from build123d import *

# Parameters (mm, degrees)
SKETCH251_AS_DRAWN_R                 = 1
EXTRUDE052_DEPTH                     = 1
EXTRUDE052_ONTO_SKETCH251_ROLL_ANGLE = 90
SKETCH249_AS_DRAWN_R                 = 2
EXTRUDE051_DEPTH                     = 1
EXTRUDE051_ONTO_SKETCH249_ROLL_ANGLE = 90
EXTRUDE047_DEPTH                     = 31
EXTRUDE047_ONTO_SKETCH246_ROLL_ANGLE = 90
CHAMFER_SIZE                         = 1
EXTRUDE046_DEPTH                     = 32
EXTRUDE046_ONTO_SKETCH244_ROLL_ANGLE = 90
FILLET_R                             = 1
SKETCH248_AS_DRAWN_R                 = 2
EXTRUDE050_DEPTH                     = 2
EXTRUDE050_ONTO_SKETCH248_ROLL_ANGLE = 90
SKETCH247_AS_DRAWN_R                 = 3
EXTRUDE049_DEPTH                     = 2
EXTRUDE049_ONTO_SKETCH247_ROLL_ANGLE = 90
FILLET001_R                          = 0.5


with BuildPart() as extrude052:
    # Sketch251 as drawn → Extrude052 (new)
    with BuildSketch(Plane.XY):
        with Locations((4.5, 0)):
            Circle(SKETCH251_AS_DRAWN_R)
        with Locations((-7.5, 0)):
            Circle(SKETCH251_AS_DRAWN_R)
        with Locations((-1.5, 5)):
            Circle(SKETCH251_AS_DRAWN_R)
    extrude(amount=-EXTRUDE052_DEPTH)


with BuildPart() as extrude052_1:
    # Extrude052 onto Sketch251 roll: moved
    add(extrude052.part.rotate(Axis((0, 0, 0), (1, 0, 0)), EXTRUDE052_ONTO_SKETCH251_ROLL_ANGLE))


with BuildPart() as extrude052_2:
    # Extrude052 onto Sketch251 placement: moved
    add(extrude052_1.part.moved(Location((1.5, 31, 0))))


with BuildPart() as extrude051:
    # Sketch249 as drawn → Extrude051 (new)
    with BuildSketch(Plane.XY):
        Circle(SKETCH249_AS_DRAWN_R)
    extrude(amount=-EXTRUDE051_DEPTH)


with BuildPart() as extrude051_1:
    # Extrude051 onto Sketch249 roll: moved
    add(extrude051.part.rotate(Axis((0, 0, 0), (1, 0, 0)), EXTRUDE051_ONTO_SKETCH249_ROLL_ANGLE))


with BuildPart() as extrude051_2:
    # Extrude051 onto Sketch249 placement: moved
    add(extrude051_1.part.moved(Location((0, 31, 0))))


with BuildPart() as chamfer_body:
    # Sketch246 as drawn → Extrude047 (new)
    with BuildSketch(Plane.XY):
        with BuildLine():
            Line((-6.5, 7.250002), (6.499997, 7.250002))
            ThreePointArc((6.499997, -7.250002), (9.737171, 0), (6.499997, 7.250002))
            Line((-6.5, -7.250002), (6.499997, -7.250002))
            ThreePointArc((-6.5, 7.250002), (-9.737172, 0), (-6.5, -7.250002))
        make_face()
    extrude(amount=-EXTRUDE047_DEPTH)


with BuildPart() as chamfer_body_1:
    # Extrude047 onto Sketch246 roll: moved
    add(chamfer_body.part.rotate(Axis((0, 0, 0), (1, 0, 0)), EXTRUDE047_ONTO_SKETCH246_ROLL_ANGLE))


with BuildPart() as chamfer_body_2:
    # Extrude047 onto Sketch246 placement: moved
    add(chamfer_body_1.part)

    # Chamfer
    chamfer_edges = [chamfer_body_2.edges().sort_by_distance(p)[0] for p in [
        (-1e-06, 31, 7.250002),
        (9.737171, 31, 0),
        (-1e-06, 31, -7.250002),
        (-9.737172, 31, 0),
    ]]
    chamfer(chamfer_edges, length=CHAMFER_SIZE)


with BuildPart() as cut032:
    # Sketch244 as drawn → Extrude046 (new)
    with BuildSketch(Plane.XY):
        with BuildLine():
            Line((-6.5, 7.499998), (6.499997, 7.499998))
            ThreePointArc((6.499997, -7.499998), (9.924714, 0), (6.499997, 7.499998))
            Line((-6.5, -7.499998), (6.499997, -7.499998))
            ThreePointArc((-6.5, 7.499998), (-9.924715, 0), (-6.5, -7.499998))
        make_face()
    extrude(amount=-EXTRUDE046_DEPTH)


with BuildPart() as cut032_1:
    # Extrude046 onto Sketch244 roll: moved
    add(cut032.part.rotate(Axis((0, 0, 0), (1, 0, 0)), EXTRUDE046_ONTO_SKETCH244_ROLL_ANGLE))


with BuildPart() as cut032_2:
    # Extrude046 onto Sketch244 placement: moved
    add(cut032_1.part)

    # Fillet
    fillet_edges = [cut032_2.edges().sort_by_distance(p)[0] for p in [
        (-1e-06, 32, 7.499998),
        (9.924714, 32, 0),
        (-1e-06, 32, -7.499998),
        (-9.924715, 32, 0),
    ]]
    fillet(fillet_edges, radius=FILLET_R)

    # Cut029: cut Chamfer body
    add(chamfer_body_2.part, mode=Mode.SUBTRACT)

    # Cut031: cut Extrude051
    add(extrude051_2.part, mode=Mode.SUBTRACT)

    # Cut032: cut Extrude052
    add(extrude052_2.part, mode=Mode.SUBTRACT)


with BuildPart() as extrude050:
    # Sketch248 as drawn → Extrude050 (new)
    with BuildSketch(Plane.XY):
        Circle(SKETCH248_AS_DRAWN_R)
    extrude(amount=-EXTRUDE050_DEPTH)


with BuildPart() as extrude050_1:
    # Extrude050 onto Sketch248 roll: moved
    add(extrude050.part.rotate(Axis((0, 0, 0), (1, 0, 0)), EXTRUDE050_ONTO_SKETCH248_ROLL_ANGLE))


with BuildPart() as extrude050_2:
    # Extrude050 onto Sketch248 placement: moved
    add(extrude050_1.part.moved(Location((0, 34, 0))))


with BuildPart() as extrude050_3:
    # Extrude050 placement: moved
    add(extrude050_2.part.moved(Location((0, -2, 0))))


with BuildPart() as fusion017:
    # Sketch247 as drawn → Extrude049 (new)
    with BuildSketch(Plane.XY):
        Circle(SKETCH247_AS_DRAWN_R)
    extrude(amount=-EXTRUDE049_DEPTH)


with BuildPart() as fusion017_1:
    # Extrude049 onto Sketch247 roll: moved
    add(fusion017.part.rotate(Axis((0, 0, 0), (1, 0, 0)), EXTRUDE049_ONTO_SKETCH247_ROLL_ANGLE))


with BuildPart() as fusion017_2:
    # Extrude049 onto Sketch247 placement: moved
    add(fusion017_1.part.moved(Location((0, 32, 0))))

    # Fillet001
    fillet001_edges = [fusion017_2.edges().sort_by_distance(p)[0] for p in [
        (-3, 34, 0),
    ]]
    fillet(fillet001_edges, radius=FILLET001_R)

    # Cut030: cut Extrude050
    add(extrude050_3.part, mode=Mode.SUBTRACT)

    # Fusion017: union Cut032
    add(cut032_2.part)


solid = fusion017_2.part
Could you check a few things on this model? Use its own coordinates, in mm. A direction names the side the tool comes from. Give positions to 0.01 mm unless a question says otherwise; leave off trailing zeros. Order: outer loops, then holes, each group sorted by start corner. A loop starts at its lowest first (then second) coordinate and runs counter-clockwise, first axis right, second up. Notation, with made-up numbers: (80.5, 52.5) - (91.5, 52.5) arc R19 cw to (91.5, 77.5) - close; hole circle Ø1 at (85, -33). An arc over 180 degrees is marked (long way). Return JSON: item names as keys, results as strings. Group by question number.
Q1. Suppose I cut it at A-A, the plane z = 0. State how many separate pieces and enclosed holes the cut face has, and give its area (3 significant figures).
Q2. Suppose I cut it at C-C, the plane y = 4.5. Please give me the cut outline in (x, z).
Q3. Suppose I cut it at B-B, the plane x = 0. Please give me the cut outline in (y, z), and give its area (3 significant figures).
Q4. Which directions (+Z, -Z, +X, -X, +Y, -Y) give clear straight access to the entire face, cutting with the end or side of a thin tool? Please do faces 4 (the face through (-3, 33, 0)), 5 (the face through (0, 15, -7.25)), 6 (the face through (0, 15, 7.5)).
Q5. Suppose I cut it at D-D, the plane x = 4.25. Please give me the cut outline in (y, z).
Q6. Please list where these lines run through material, in increasing order: line 1 along Z through (x, y) = (-6, 12.5); line 2 along Y through (x, z) = (-2.25, 2.5). Write a range as [from, to].
Q7. Will these pins go through, and if not, where does the flat tip stop? pin 1 Ø8 at (x, z) = (-3, 5.5) entering from +Y; pin 2 Ø6.5 at (x, z) = (0, 0) entering from -Y; pin 3 Ø6 at (y, z) = (8, 4.5) entering from -X.
Q8. Thinking about a two-plate mould opening in Z: for faces 1 (the face through (-1, 34, 2)), 2 (the face through (-2, 31, -1)), 3 (the face through (0.091, 31.699, 7.215)), which applies, pulls with the +Z half, pulls with the -Z half, needs draft (parallel to the pull), parting line crosses it, or undercut?
Resolved:
{
 "1": {"separate pieces": "4", "enclosed holes": "0", "area": "27.9 mm2"},
 "2": {"outline": "(-6.5, -7.5) - (6.5, -7.5) arc R9.92 ccw to (6.5, 7.5) - (-6.5, 7.5) arc R9.92 ccw to start; hole (-6.5, -7.25) - (6.5, -7.25) arc R9.74 ccw to (6.5, 7.25) - (-6.5, 7.25) arc R9.74 ccw to start"},
 "3": {"outline": "(0, -7.5) - (31, -7.5) arc R1 ccw to (32, -6.5) - (32, -3) - (33.5, -3) arc R0.5 ccw to (34, -2.5) - (34, -2) - (31, -2) - (31, -6.25) - (30, -7.25) - (0, -7.25) - close; (0, 7.25) - (30, 7.25) - (31, 6.25) - (31, 6) - (32, 6) - (32, 6.5) arc R1 ccw to (31, 7.5) - (0, 7.5) - close; (31, 2) - (34, 2) - (34, 2.5) arc R0.5 ccw to (33.5, 3) - (32, 3) - (32, 4) - (31, 4) - close", "area": "29.0 mm2"},
 "4": {"face 4": "+Y", "face 5": "-Y", "face 6": "+Z, +X, -X, +Y, -Y"},
 "5": {"outline": "(0, -7.5) - (31, -7.5) arc R1 ccw to (32, -6.5) - (32, 6.5) arc R1 ccw to (31, 7.5) - (0, 7.5) - (0, 7.25) - (30, 7.25) - (31, 6.25) - (31, -6.25) - (30, -7.25) - (0, -7.25) - close"},
 "6": {"line 1": "z = [-7.5, -7.25], [7.25, 7.5]", "line 2": "y = [31, 32]"},
 "7": {"pin 1": "stops at y = 34", "pin 2": "stops at y = 31", "pin 3": "stops at x = -9.81"},
 "8": {"face 1": "needs draft", "face 2": "undercut", "face 3": "pulls with the +Z half"}
}
